Check sheet for the modelled part. Datum: model origin and axes. Units: mm. Face numbers are marked on the shaded views. A direction names the side the tool comes from. Coordinates: 2 decimals unless noted, no trailing zeros. Write each loop counter-clockwise with the first axis right and the second up, starting at its lowest first coordinate (ties: lowest second). Pieces come first, ordered by that corner, then holes. Notation, with made-up numbers: (54.25, 0) -> (87.25, 0) arc R13 ccw to (87.25, 20) -> close; hole circle Ø7 at (56.25, 39). An arc over 180 degrees is marked (long way). Put each result on its own line as item: value.
```python
from build123d import *

# Parameters (mm, degrees)
SKETCH_1_R          = 4
SKETCH_1_R_2        = 1.75
EXTRUDE_1_DEPTH     = 3
EXTRUDE_2_DEPTH     = 26
CUT_EXTRUDE_1_DEPTH = 55.571054599
EXTRUDE_4_DEPTH     = 3


with BuildPart() as part:
    # 草图1 → 凸台-拉伸1 (new body)
    with BuildSketch(Plane(origin=(0, 0, 0), x_dir=(1, 0, 0), z_dir=(0, 1, 0))):
        with BuildLine():
            Line((-13, 0), (-13, -30))
            Line((-13, -30), (13, -30))
            Line((13, -30), (13, 0))
            ThreePointArc((13, 0), (0, 13), (-13, 0))
        make_face()
        with Locations(Location((0, 0, 0), (0, 0, 270))):
            Circle(SKETCH_1_R, mode=Mode.SUBTRACT)
        with Locations(Location((8.5, 0, 0), (0, 0, 270))):
            Circle(SKETCH_1_R_2, mode=Mode.SUBTRACT)
        with Locations(Location((-8.5, 0, 0), (0, 0, 270))):
            Circle(SKETCH_1_R_2, mode=Mode.SUBTRACT)
    extrude(amount=EXTRUDE_1_DEPTH)

    # 草图4 → 凸台-拉伸2 (add)
    with BuildSketch(Plane(origin=(13, 0, 0), x_dir=(0, 0, -1), z_dir=(1, 0, 0))):
        Polygon((-30, 3), (-30, 31), (-45, 31), (-45, 28), (-33, 28), (-33, 0), (-30, 0), align=None)
    extrude(amount=-EXTRUDE_2_DEPTH)

    # 草图6 → 切除-拉伸1 (cut, through all)
    with BuildSketch(Plane.XZ.offset(-28)):
        with BuildLine():
            ThreePointArc((9.25, 42), (7.5, 43.75), (5.75, 42))
            Line((5.75, 42), (7.5, 42))
            Line((7.5, 42), (7.5, 40.25))
            ThreePointArc((7.5, 40.25), (8.737436867, 40.762563133), (9.25, 42))
        make_face()
        with BuildLine():
            Line((7.5, 42), (5.75, 42))
            ThreePointArc((5.75, 42), (6.262563133, 40.762563133), (7.5, 40.25))
            Line((7.5, 40.25), (7.5, 42))
        make_face()
        with BuildLine():
            ThreePointArc((1.75, 37), (0, 38.75), (-1.75, 37))
            Line((-1.75, 37), (1.75, 37))
        make_face()
        with BuildLine():
            Line((1.75, 37), (-1.75, 37))
            ThreePointArc((-1.75, 37), (0, 35.25), (1.75, 37))
        make_face()
        with BuildLine():
            Line((-7.5, 40.25), (-7.5, 42))
            Line((-7.5, 42), (-5.75, 42))
            ThreePointArc((-5.75, 42), (-8.737436867, 43.237436867), (-7.5, 40.25))
        make_face()
        with BuildLine():
            Line((-5.75, 42), (-7.5, 42))
            Line((-7.5, 42), (-7.5, 40.25))
            ThreePointArc((-7.5, 40.25), (-6.262563133, 40.762563133), (-5.75, 42))
        make_face()
    extrude(amount=-CUT_EXTRUDE_1_DEPTH, mode=Mode.SUBTRACT)

    # 草图7 → 凸台-拉伸4 (add)
    with BuildSketch(Plane.XZ):
        with BuildLine():
            ThreePointArc((-6.7e-08, -13), (-9.192388179, -9.192388132), (-13, 0))
            Line((-13, 0), (-13, -13))
            Line((-13, -13), (-6.7e-08, -13))
        make_face()
        with BuildLine():
            ThreePointArc((13, 0), (9.192388132, -9.192388179), (-6.7e-08, -13))
            Line((-6.7e-08, -13), (13, -13))
            Line((13, -13), (13, 0))
        make_face()
    extrude(amount=-EXTRUDE_4_DEPTH)


solid = part.part
```
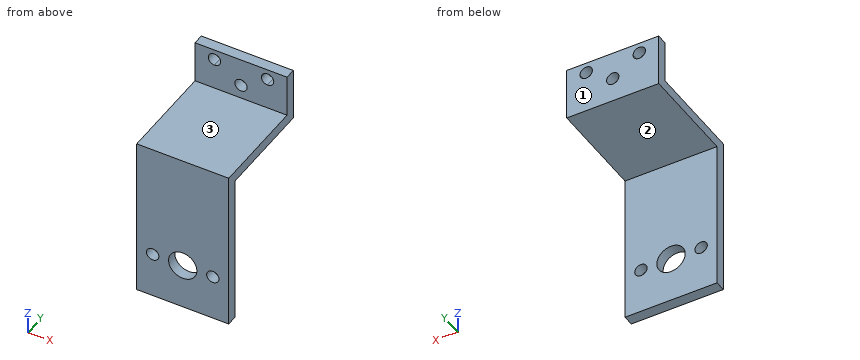
Q1. Cross-section at D-D (y = 26). Record the cut outline in (x, z).
Recorded:
outline: (-13, 30) -> (13, 30) -> (13, 33) -> (-13, 33) -> close
Q2. Tool access check on the marked faces 1, 2 and 3. Record the directions out of +Z, -Z, +X, -X, +Y, -Y that give a thin tool (end or side, any length) a straight path to the whole face; none if there is none.
Recorded:
face 1: +Z, -Z, +X, -X, +Y
face 2: -Z, +X, -X, +Y
face 3: +Z, +X, -X, -Y
Q3. Cross-section at A-A (z = 0). Record the cut outline in (x, y).
Recorded:
outline: (-13, 0) -> (-10.25, 0) -> (-10.25, 3) -> (-13, 3) -> close; (-6.75, 0) -> (-4, 0) -> (-4, 3) -> (-6.75, 3) -> close; (4, 0) -> (6.75, 0) -> (6.75, 3) -> (4, 3) -> close; (10.25, 0) -> (13, 0) -> (13, 3) -> (10.25, 3) -> close
Q4. Cross-section at C-C (x = -11). Record the cut outline in (y, z), plus the area to 3 significant figures.
Recorded:
outline: (0, -13) -> (3, -13) -> (3, 30) -> (31, 30) -> (31, 45) -> (28, 45) -> (28, 33) -> (0, 33) -> close
area: 258 mm2
Q5. Depth check by flat-ended pin: P1, Ø3.5, axis at x = 0.5, z = 39.5, coming from the -Y side; P2, Ø4.5, axis at x = 8.5, z = 0, coming from the +Y side; P3, Ø1, axis at x = -6.5, y = 19.5, coming from the +Z side; P4, Ø10, axis at y = 10.5, z = -2.5, coming from the +X side. Enter the tip coordinate at first touch or a pass-through.
Recorded:
P1: stops at y = 28
P2: stops at y = 3
P3: stops at z = 33
P4: passes through
Q6. Material ranges on line 1 along X through (y, z) = (30.2, 42); line 2 along X through (y, z) = (1.95, 0); line 3 along Y through (x, z) = (10.5, 38), recorded low to high.
Recorded:
line 1: x = -13 to -9.25, -5.75 to 5.75, 9.25 to 13
line 2: x = -13 to -10.25, -6.75 to -4, 4 to 6.75, 10.25 to 13
line 3: y = 28 to 31
Q7. Cross-section at B-B (x = 0). Record the cut outline in (y, z).
Recorded:
outline: (0, -13) -> (3, -13) -> (3, -4) -> (0, -4) -> close; (0, 4) -> (3, 4) -> (3, 30) -> (31, 30) -> (31, 35.25) -> (28, 35.25) -> (28, 33) -> (0, 33) -> close; (28, 38.75) -> (31, 38.75) -> (31, 45) -> (28, 45) -> close
